Source: CAD feature listing. Evaluate the final solid. Frame: model axes, mm. Coordinates: 2 decimals unless noted, no trailing zeros. Order: outer loops, then holes, each group sorted by start corner. A loop starts at its lowest first (then second) coordinate and runs counter-clockwise, first axis right, second up. Notation, with made-up numbers: (85, 9.5) -> (135, 9.5) arc R15 cw to (135, 27.5) -> close; hole circle Ø1 at (39, 34.25). An arc over 180 degrees is marked (long way). Write item = value, one per line. Start each with the question number.
Item 1: Contact query for flat-ended pins moving along their axis: pin 1 (0.5 mm diameter, centred on x = 2.5, y = -4, fed in from +Z); pin 2 (1.4 mm diameter, centred on x = 2, z = -2, fed in from -Y); pin 3 (0.5 mm diameter, centred on x = 2, z = -32, fed in from +Y); pin 4 (10 mm diameter, centred on y = -9, z = -26, fed in from +X). Output: stop coordinate, or through.
Item 2: Ray query, line 1 along Y through (x, z) = (2.4, 30); line 2 along Z through (x, y) = (3.6, -11.5); line 3 along Z through (x, y) = (3.75, -8.5). Return the intervals inside material, ascending. Write a range as [from, to].
Item 3: Section query B-B (z = 27). Output: boundary loops of the cut face in (x, y).
Item 4: Section query A-A (x = 2.6). Output: boundary loops of the cut face in (y, z), then the cut area to 3 significant figures.
Item 5: Section query C-C (y = -16). Output: boundary loops of the cut face in (x, z), then the cut area to 3 significant figures.
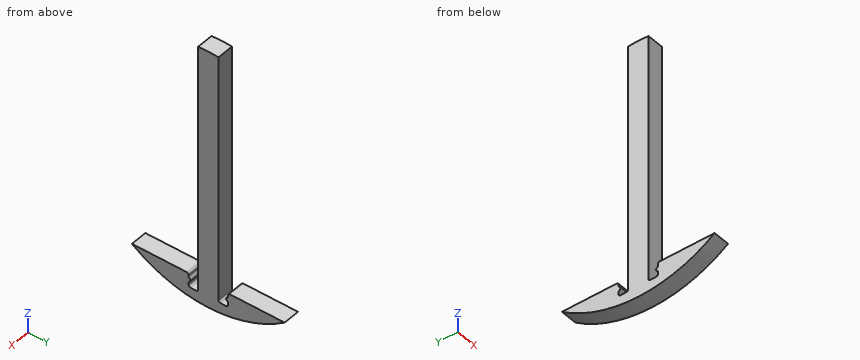
```python
from build123d import *

# Parameters (mm, degrees)
SKETCH1_R           = 35.75
BOSS_EXTRUDE1_DEPTH = 4.6
CUT_EXTRUDE1_DEPTH  = 51.766967607
FILLET1_R           = 0.5
FILLET2_R           = 0.5


with BuildPart() as part:
    # Sketch1 → Boss-Extrude1 (new body)
    with BuildSketch(Plane(origin=(0, 0, 0), x_dir=(0, 0, -1), z_dir=(1, 0, 0))):
        Circle(SKETCH1_R)
    extrude(amount=BOSS_EXTRUDE1_DEPTH)

    # Sketch2 → Cut-Extrude1 (cut, through all)
    with BuildSketch(Plane(origin=(4.6, 0, 0), x_dir=(0, 0, -1), z_dir=(1, 0, 0))):
        with BuildLine():
            Line((28.95, 5.4), (28.95, 20.975223479))
            ThreePointArc((28.95, 20.975223479), (-9.683714035, 34.41348838), (-35.640180976, 2.8))
            Line((-35.640180976, 2.8), (28.95, 2.8))
            Line((28.95, 2.8), (28.95, 5.4))
        make_face()
        with BuildLine():
            ThreePointArc((-35.640180976, -2.8), (-9.683714035, -34.41348838), (28.95, -20.975223479))
            Line((28.95, -20.975223479), (28.95, -5.4))
            Line((28.95, -5.4), (28.95, -2.8))
            Line((28.95, -2.8), (-35.640180976, -2.8))
        make_face()
        with BuildLine():
            Line((28.95, 2.8), (32.75, 2.8))
            Line((32.75, 2.8), (32.75, 5.4))
            Line((32.75, 5.4), (31.25, 5.4))
            ThreePointArc((31.25, 5.4), (30.75, 4.9), (30.25, 5.4))
            Line((30.25, 5.4), (28.95, 5.4))
            Line((28.95, 5.4), (28.95, 2.8))
        make_face()
        with BuildLine():
            Line((32.75, -5.4), (32.75, -2.8))
            Line((32.75, -2.8), (28.95, -2.8))
            Line((28.95, -2.8), (28.95, -5.4))
            Line((28.95, -5.4), (30.25, -5.4))
            ThreePointArc((30.25, -5.4), (30.75, -4.9), (31.25, -5.4))
            Line((31.25, -5.4), (32.75, -5.4))
        make_face()
    extrude(amount=-CUT_EXTRUDE1_DEPTH, mode=Mode.SUBTRACT)

    # Fillet1
    fillet1_edges = [part.edges().sort_by_distance(p)[0] for p in [
        (2.3, 5.4, -28.95),
        (2.3, 5.4, -32.75),
        (2.3, 2.8, -32.75),
        (2.3, -5.4, -28.95),
        (2.3, -2.8, -32.75),
        (2.3, -5.4, -32.75),
    ]]
    fillet(fillet1_edges, radius=FILLET1_R)

    # Fillet2
    fillet2_edges = [part.edges().sort_by_distance(p)[0] for p in [
        (2.3, 5.4, -30.25),
        (2.3, 5.4, -31.25),
        (2.3, -5.4, -31.25),
        (2.3, -5.4, -30.25),
    ]]
    fillet(fillet2_edges, radius=FILLET2_R)


solid = part.part
```
Computed:
q1.pin_1 = -32.75
q1.pin_2 = -2.8
q1.pin_3 = 16.43
q1.pin_4 = 4.6
q2.line_1 = [-2.8, 2.8]
q2.line_2 = [-33.85, -28.95]
q2.line_3 = [-34.72, -28.95]
q3.outline = (0, -2.8) -> (4.6, -2.8) -> (4.6, 2.8) -> (0, 2.8) -> close
q4.outline = (-20.98, -28.95) arc R35.75 ccw to (20.98, -28.95) -> (5.9, -28.95) arc R0.5 ccw to (5.4, -29.45) -> (5.4, -29.88) arc R0.5 cw to (5.15, -30.32) arc R0.5 ccw to (5.15, -31.18) arc R0.5 cw to (5.4, -31.62) -> (5.4, -32.25) arc R0.5 cw to (4.9, -32.75) -> (3.3, -32.75) arc R0.5 cw to (2.8, -32.25) -> (2.8, 35.64) arc R35.75 ccw to (-2.8, 35.64) -> (-2.8, -32.25) arc R0.5 cw to (-3.3, -32.75) -> (-4.9, -32.75) arc R0.5 cw to (-5.4, -32.25) -> (-5.4, -31.62) arc R0.5 cw to (-5.15, -31.18) arc R0.5 ccw to (-5.15, -30.32) arc R0.5 cw to (-5.4, -29.88) -> (-5.4, -29.45) arc R0.5 ccw to (-5.9, -28.95) -> close
q4.area = 537 mm^2
q5.outline = (0, -31.97) -> (4.6, -31.97) -> (4.6, -28.95) -> (0, -28.95) -> close
q5.area = 13.9 mm^2
